Model file for the job. Use its own axes, mm. Coordinates: 2 decimals unless noted, no trailing zeros. Order: outer loops, then holes, each group sorted by start corner. A loop starts at its lowest first (then second) coordinate and runs counter-clockwise, first axis right, second up.
Autodesk Inventor part; units mm, degrees
ref_plane "YZ Plane" through (0, 0, 0) normal (1, 0, 0) x (0, 1, 0)
ref_plane "XZ Plane" through (0, 0, 0) normal (0, 1, 0) x (-1, 0, 0)
ref_plane "XY Plane" through (0, 0, 0) normal (0, 0, 1) x (1, 0, 0)
sketch "Sketch1" plane through (0, 0, 0) normal (1, 0, 0) x (0, 1, 0)
  line L0 (0, 0) -> (-50.8, 0)
  line L1 (-50.8, 0) -> (-50.8, -25.4)
  line L2 (-50.8, -25.4) -> (0, -25.4)
  line L3 (0, -25.4) -> (0, 0)
  line L4 (-3.175, -3.175) -> (-47.625, -3.175)
  line L5 (-47.625, -3.175) -> (-47.625, -22.225)
  line L6 (-47.625, -22.225) -> (-3.175, -22.225)
  line L7 (-3.175, -22.225) -> (-3.175, -3.175)
  dimension "d0" = 50.8
  dimension "d1" = 25.4
  dimension "d2" = 3.175
extrude "Extrusion1" add sketch "Sketch1" along normal blind 127
sketch "Sketch2" plane through (0, -50.8, 0) normal (0, 0, 1) x (1, 0, 0)
  line L0 (0, 50.8) -> (0, 0)
  line L1 (0, 0) -> (127, 0)
  line L2 (127, 50.8) -> (127, 0)
  line L3 (0, 50.8) -> (127, 50.8)
  circle A0 centre (63.5, 6.0325) radius 3.175
  circle A1 centre (63.5, 33.3375) radius 6.35
  circle A2 centre (63.5, 33.3375) radius 14.2875
  circle A3 centre (63.5, 33.3375) radius 7.62
  circle A4 centre (63.5, 33.3375) radius 15.875
  line L4 (0, 47.625) -> (127, 47.625)
  dimension "d5" = 6.35
  dimension "d6" = 12.7
  dimension "d9" = 28.575
  dimension "d10" = 15.24
  dimension "d11" = 31.75
  dimension "d12" = 14.2875
  dimension "d13" = 16.51
extrude "Extrusion2" cut sketch "Sketch2" against normal blind 127 contours A2 | A0 | A1 | A3
sketch "Sketch3" plane through (0, -50.8, -25.4) normal (0, 0, -1) x (-1, 0, 0)
  circle A0 centre (-63.5, 33.3375) radius 14.2875
  circle A1 centre (-63.5, 6.0325) radius 3.175
  line L0 (0, 0) -> (0, 50.8)
  line L1 (0, 50.8) -> (-127, 50.8)
  line L2 (-127, 0) -> (-127, 50.8)
  line L3 (0, 0) -> (-127, 0)
  point P0 (-38.1, 6.0325)
  point P1 (-12.7, 6.0325)
  point P2 (-88.9, 6.0325)
  point P3 (-114.3, 6.0325)
  dimension "d16" = 25.4
  dimension "d17" = 25.4
  dimension "d18" = 25.4
  dimension "d19" = 25.4
hole "Hole1" at (38.1, -44.7675, -25.4) at (12.7, -44.7675, -25.4) at (88.9, -44.7675, -25.4) at (114.3, -44.7675, -25.4) direction (0, 0, 1) diameter 6.35 end through all
sketch "Sketch4" plane through (0, 0, 0) normal (-1, 0, 0) x (0, 0, 1)
  line L0 (0, 0) -> (-25.4, 0)
  line L1 (-25.4, 0) -> (-25.4, -101.6)
  line L2 (-25.4, -101.6) -> (0, -101.6)
  line L3 (0, -101.6) -> (0, 0)
  line L4 (-3.175, -98.425) -> (-22.225, -98.425)
  line L5 (-22.225, -98.425) -> (-22.225, -3.175)
  line L6 (-22.225, -3.175) -> (-3.175, -3.175)
  line L7 (-3.175, -3.175) -> (-3.175, -98.425)
  line L8 (-3.175, -47.625) -> (-3.175, -3.175)
  line L9 (-22.225, -61.2712) -> (-3.175, -61.2712)
  line L10 (-3.175, -61.2712) -> (-3.175, -33.0722)
  line L11 (-3.175, -33.0722) -> (-22.225, -33.0722)
  line L12 (-22.225, -33.0722) -> (-22.225, -61.2712)
  line L13 (-22.225, -3.175) -> (-3.175, -3.175)
  line L14 (-3.175, -3.175) -> (-3.175, -47.625)
  line L15 (-3.175, -47.625) -> (-22.225, -47.625)
  line L16 (-22.225, -47.625) -> (-22.225, -3.175)
  line L17 (0, 0) -> (0, -50.8)
  line L18 (-25.4, 0) -> (0, 0)
  line L19 (-25.4, -50.8) -> (-25.4, 0)
  line L20 (0, -50.8) -> (-25.4, -50.8)
  line L21 (-25.4, -50.8) -> (-22.225, -50.8)
  line L22 (0, -50.8) -> (-25.4, -50.8)
  line L23 (-3.175, -50.8) -> (0, -50.8)
  dimension "d27" = 25.4
  dimension "d28" = 101.6
  dimension "d29" = 3.175
extrude "Extrusion3" cut sketch "Sketch4" against normal blind 127 contours L20 L5 L15 L7 | L7 L9 L5 L20 | L15 L5 L11 L7
extrude "Extrusion4" add sketch "Sketch4" against normal blind 127 contours L3 L2 L1 L20 L5 L4 L7
sketch "Sketch5" plane through (127, 0, -25.4) normal (0, 0, -1) x (-1, 0, 0)
  line L0 (-34.6309, 15.7259) -> (-18.4019, -170.3675)
  line L1 (-18.4019, -170.3675) -> (166.6096, -150.8926)
  line L2 (166.6096, -150.8926) -> (166.6096, -41.3464)
  line L3 (166.6096, -41.3464) -> (138.7497, 15.7259)
  line L4 (138.7497, 15.7259) -> (-34.6309, 15.7259)
  point P0 (127, 0)
extrude "Extrusion5" cut sketch "Sketch5" against normal blind 22.225
sketch "Sketch6" plane through (0, 0, 0) normal (0, 0, 1) x (1, 0, 0)
  circle A0 centre (12.7, -44.7675) radius 3.175
  line L0 (12.7, -44.7675) -> (0, -44.7675)
  line L1 (0, 0) -> (0, -101.6)
  line L2 (0, -44.7675) -> (0, -57.4675)
  line L3 (0, -57.4675) -> (127, -57.4675)
  line L4 (127, 0) -> (127, -101.6)
  line L5 (12.7, -44.7675) -> (127, -44.7675)
  line L6 (127, -44.7675) -> (127, -57.4675)
  line L7 (127, -57.4675) -> (144.4596, -106.2687)
  line L8 (144.4596, -106.2687) -> (111.8065, -115.7811)
  line L9 (111.8065, -115.7811) -> (9.525, -135.9925)
  line L10 (9.525, -135.9925) -> (-52.3397, -101.6)
  line L11 (-52.3397, -101.6) -> (0, -57.4675)
  dimension "d36" = 12.7
  dimension "d37" = 12.7
extrude "Extrusion6" cut sketch "Sketch6" against normal blind 22.225 contours L7 L8 L9 L10 L11 L3
sketch "Sketch7" plane through (0, -57.4675, 0) normal (0, -1, 0) x (1, 0, 0)
  line L0 (127, -3.175) -> (127, 0)
  line L1 (0, 0) -> (127, 0)
  line L2 (127, 0) -> (0, 0)
  line L3 (0, 0) -> (0, -3.175)
  line L4 (0, -3.175) -> (127, -3.175)
  line L5 (127, -3.175) -> (0, -3.175)
sketch "Sketch8" plane through (0, 0, 0) normal (0, 1, 0) x (1, 0, 0)
  line L0 (0, 0) -> (0, 3.175)
  line L1 (0, 3.175) -> (127, 3.175)
  line L2 (127, 3.175) -> (127, 0)
  line L3 (127, 0) -> (0, 0)
extrude "Extrusion8" add sketch "Sketch8" along normal blind 3.1623
sketch "Sketch9" plane through (127, 0, 0) normal (1, 0, 0) x (0, 0, -1)
  line L0 (0, 3.1623) -> (3.175, 3.1623)
  line L1 (3.175, 3.1623) -> (0, 3.1623)
  line L2 (3.175, 3.1623) -> (3.175, -57.4675)
  line L3 (3.175, -57.4675) -> (0, -57.4675)
  line L4 (0, -57.4675) -> (3.175, -57.4675)
  line L5 (0, -57.4675) -> (0, 3.1623)
  point P0 (0, 0)
extrude "Extrusion9" cut sketch "Sketch9" against normal blind 25.4
sketch "Sketch10" plane through (0, 0, 0) normal (-1, 0, 0) x (0, 0, 1)
  line L0 (0, 3.1623) -> (0, -57.4675)
  line L1 (0, -57.4675) -> (-3.175, -57.4675)
  line L2 (-3.175, -57.4675) -> (-3.175, 3.1623)
  line L3 (-3.175, 3.1623) -> (-3.175, -57.4675)
  line L4 (-3.175, 3.1623) -> (0, 3.1623)
  point P0 (0, 0)
extrude "Extrusion10" cut sketch "Sketch10" against normal blind 25.4
properties part number "Elevator Shaft Mounts"
Q1. Mould opens along Y. For faces 1 (the face through (63, -57.468, -2)), 2 (the face through (101.6, -27, -2)), 3 (the face through (49.226, -16.834, -1.565)), 4 (the face through (66.528, -43.814, -1.565)) say: pulls with the +Y half, pulls with the -Y half, needs draft (parallel to the pull), parting line crosses it, or undercut.
Established:
face 1: pulls with the -Y half
face 2: needs draft
face 3: undercut
face 4: undercut
Q2. Cut at A-A, the plane x = 63.5. Count the separate pieces of the cut face and the enclosed holes in it, plus the area to 3 significant figures.
Established:
separate pieces: 3
enclosed holes: 0
area: 81.6 mm2
Q3. Cut at D-D, the plane y = -21. List the corners of the cut face in (x, z) (3 decimals), plus the area to 3 significant figures.
Established:
outline: (25.4, -3.175) - (49.657, -3.175) - (49.657, 0) - (25.4, 0) - close; (77.343, -3.175) - (101.6, -3.175) - (101.6, 0) - (77.343, 0) - close
area: 154 mm2
Q4. Drop a flat-ended pin along its axis: P1, Ø5, axis at x = 38.1, y = -44.77, coming from the +Z side. Give the stop position or say it passes through.
Established:
P1: passes through
Q5. Cut at B-B, the plane x = 38.1. List the corners of the cut face in (y, z) (1 decimal).
Established:
outline: (-57.5, -3.2) - (-47.9, -3.2) - (-47.9, 0) - (-57.5, 0) - close; (-41.6, -3.2) - (3.2, -3.2) - (3.2, 0) - (-41.6, 0) - close
Q6. Probe line 1 (X direction, y = -45, z = -2.45); line 2 (Y direction, x = 38.1, z = -2.5); line 3 (X direction, y = -45.5, z = -1.85). List the from-to ranges inside material, lowest first.
Established:
line 1: x = 25.4 to 34.93, 41.27 to 60.33, 66.67 to 85.73, 92.07 to 101.6
line 2: y = -57.47 to -47.94, -41.59 to 3.16
line 3: x = 25.4 to 35.01, 41.19 to 60.41, 66.59 to 85.81, 91.99 to 101.6
